Autodesk Inventor part; units mm, degrees
ref_plane "Work Plane1" through (196, 42, -75) normal (0, 0, -1) x (-1, 0, 0)
ref_plane "YZ Plane" through (0, 0, 0) normal (1, 0, 0) x (0, 1, 0)
ref_plane "XZ Plane" through (0, 0, 0) normal (0, 1, 0) x (-1, 0, 0)
sketch "Sketch4" plane through (0, 0, 0) normal (0, 0, 1) x (1, 0, 0)
  line L0 (0, 0) -> (200, 0) construction
  line L1 (0, 0) -> (200, 0) construction
  line L2 (100, 0) -> (100, 8)
  arc A0 (200, 0) -> (0, 0) centre (100, -621) ccw
  line L3 (0, 0) -> (0, 4)
  line L4 (200, 0) -> (200, 4)
  line L5 (100, 8) -> (100, 12)
  arc A1 (200, 4) -> (0, 4) centre (100, -617) ccw
  dimension "d11" = 200
  dimension "d13" = 8
  dimension "d14" = 4
  dimension "d15" = 4
extrude "Extrusion5" add sketch "Sketch4" against normal blind 150
sketch "Sketch5" plane through (0, 0, 0) normal (0, 0, 1) x (1, 0, 0)
  arc A0 (200, 4) -> (0, 4) centre (100, -617) ccw
  line L0 (100, 12) -> (100, 8)
  arc A1 (200, 0) -> (0, 0) centre (100, -621) ccw
  line L1 (0, 4) -> (200, 4)
  line L2 (200, 4) -> (200, 12)
  line L3 (200, 12) -> (0, 12)
  line L4 (0, 12) -> (0, 4)
  point P0 (200, 4)
extrude "Extrusion6" add sketch "Sketch5" against normal up to surface (150 mm away) contours A0 L3 L2 | A0 L4 L3
sketch "Sketch6" plane through (0, 12, 0) normal (0, 1, 0) x (1, 0, 0)
  line L0 (0, 0) -> (0, 150)
  line L1 (200, 0) -> (200, 150)
  line L2 (0, 150) -> (200, 150)
  line L3 (200, 150) -> (200, 0)
  line L4 (200, 0) -> (0, 0)
  line L5 (0, 0) -> (0, 150)
  line L6 (196, 4) -> (4, 4)
  line L7 (4, 4) -> (4, 146)
  line L8 (4, 146) -> (196, 146)
  line L9 (196, 146) -> (196, 4)
  dimension "d22" = 192
  dimension "d23" = 142
extrude "Extrusion7" add sketch "Sketch6" along normal blind 30
sketch "Sketch7" plane through (0, 0, 0) normal (0, 0, 1) x (1, 0, 0)
  line L0 (196, 12) -> (4, 12)
  line L1 (100, 12) -> (100, 25) construction
  circle A0 centre (100, 25) radius 13
  point P0 (0, 0)
  dimension "d26" = 13
  dimension "d27" = 26
extrude "Extrusion8" cut sketch "Sketch7" against normal up to surface (150 mm away)
sketch "Sketch8" plane through (4, 12, -4) normal (0, 1, 0) x (1, 0, 0)
  line L0 (192, 0) -> (192, 142)
  line L1 (192, 0) -> (192, 25)
  line L2 (96, 142) -> (0, 142)
  line L3 (0, 142) -> (0, 0)
  line L4 (192, 25) -> (177, 25)
  circle A0 centre (177, 25) radius 7.5
  line L5 (177, 32.5) -> (192, 32.5)
  line L6 (192, 32.5) -> (192, 17.5)
  line L7 (192, 17.5) -> (177, 17.5)
  line L8 (177, 17.5) -> (177, 32.5)
  line L9 (192, 0) -> (96, 0) construction
  line L10 (96, 0) -> (96, 71) construction
  line L11 (96, 71) -> (192, 71) construction
  line L12 (192, 71) -> (192, 0) construction
  point P0 (-4, -4)
  point P1 (177, 17.5)
  dimension "d33" = 15
  dimension "d30" = 25
  dimension "d32" = 15
extrude "Extrusion9" add sketch "Sketch8" along normal blind 20
sketch "Sketch9" plane through (4, 32, -4) normal (0, 1, 0) x (1, 0, 0)
  line L0 (192, 17.5) -> (177, 17.5)
  arc A0 (177, 32.5) -> (177, 17.5) centre (177, 25) ccw
  line L1 (177, 17.5) -> (177, 32.5)
  point P0 (-4, -4)
hole "Hole1" at (181, 32, -29) direction (0, -1, 0) diameter 6 end through all
pattern_circular "Circular Pattern1" count 2 over 360 about axis through (100, 2.6712, -75) along (0, 1, 0) of "Hole1", "Extrusion9"
ref_plane "Work Plane1" through (196, 42, -75) normal (0, 0, -1) x (-1, 0, 0)
mirror "Mirror1" about plane through (196, 42, -75) normal (0, 0, -1) of "Hole1", "Extrusion9", "Circular Pattern1"
properties part number "McCase"
Work out the finished part from the listing and answer in its coordinate system (mm). A direction names the side the tool comes from. Give positions to 0.01 mm unless a question says otherwise; leave off trailing zeros. Loops run counter-clockwise (first coordinate to the right, second up) from the corner with the lowest first, then second, coordinate; pieces in that order, holes last. Notation, with made-up numbers: (-35, 4) - (-2, 4) arc R19 cw to (-2, 34) - close; hole circle Ø3 at (-38.75, -3.75). An arc over 180 degrees is marked (long way). Answer in a Markdown table with one row per item. Add a question column.
Q1. Each of these flat-tipped pins is pushed along its axis until it touches: P1, Ø4, axis at x = 151, y = 33, coming from the +Z side; P2, Ø4.5, axis at x = 182.5, z = -123, coming from the +Y side; P3, Ø8, axis at x = 181, z = -29, coming from the -Y side; P4, Ø8, axis at x = 166, z = -44, coming from the +Y side. Where does it stop, or does it pass through?
Q2. The part is cut by section B-B (y = 25). State how many separate pieces and enclosed holes the cut face has, and give its area (3 significant figures).
Q3. The part is cut by section D-D (z = -95.5). Determine the outline of the cut face in (x, y).
Q4. The part is cut by section A-A (z = -121). Determine the outline of the cut face in (x, y).
Q5. A tool of negligible diameter and unlimited length cuts with its end or side. For faces 1 (the flat face through (188, 22, -36.5)), 2 (the cylindrical face through (20.8, 17, -31.4)), from which of +Z, -Z, +X, -X, +Y, -Y can it reach the whole face along a straight path? Write none if from no direction.
Q6. Determine the mould class of faces 3 (the flat face through (3, 42, -75)), 4 (the flat face through (101, 11, 0)), 5 (the cylindrical face through (178, 17, -29)) for opening direction Z: released by +Z, released by -Z, zero draft, split by the parting line, or undercut.
Q7. Consider line 1 along Z through (x, y) = (19, 20); line 2 along X through (y, z) = (23, -29); line 3 along Z through (x, y) = (109, 35.5). Determine where each line is inside the solid, lowest interval first.
Solution:
| question | item | result |
|---|---|---|
| 1 | P1 | stops at z = 0 |
| 1 | P2 | stops at y = 32 |
| 1 | P3 | stops at y = 2.23 |
| 1 | P4 | stops at y = 12 |
| 2 | separate pieces | 2 |
| 2 | enclosed holes | 4 |
| 2 | area | 3,670 mm² |
| 3 | outline | (0, 0) arc R629 cw to (200, 0) - (200, 42) - (196, 42) - (196, 12) - (4, 12) - (4, 42) - (0, 42) - close |
| 4 | outline | (0, 0) arc R629 cw to (16, 2.37) - (16, 32) - (4, 32) - (4, 42) - (0, 42) - close; (22, 3.15) arc R629 cw to (178, 3.15) - (178, 32) - (173.5, 32) - (173.5, 12) - (26.5, 12) - (26.5, 32) - (22, 32) - close; (184, 2.37) arc R629 cw to (200, 0) - (200, 42) - (196, 42) - (196, 32) - (184, 32) - close |
| 5 | face 1 | +Y |
| 5 | face 2 | +Y, -Y |
| 6 | face 3 | zero draft |
| 6 | face 4 | released by +Z |
| 6 | face 5 | undercut |
| 7 | line 1 | z = -150 to -146, -128.5 to -124, -118 to -113.5, -36.5 to -32, -26 to -21.5, -4 to 0 |
| 7 | line 2 | x = 0 to 16, 22 to 26.5, 173.5 to 178, 184 to 200 |
| 7 | line 3 | z = -150 to -146, -4 to 0 |
